```python
from build123d import *

# Parameters (mm, degrees)
SKETCH2_R          = 15
SKETCH2_R_2        = 8.75
M10_TAPPED_HOLE1_D = 8.5
M10_TAPPED_HOLE2_D = 8.5


with BuildPart() as part:
    # Sweep1: sweep along a path in Sketch1
    with BuildLine(Plane(origin=(0, 0, 0), x_dir=(1, 0, 0), z_dir=(0, 1, 0))) as sweep1_path:
        Line((175, 180), (175, 30))
        ThreePointArc((175, 30), (166.213203436, 8.786796564), (145, 0))
        Line((145, 0), (-145, 0))
        ThreePointArc((-145, 0), (-166.213203436, -8.786796564), (-175, -30))
        Line((-175, -30), (-175, -180))
    # Sketch2 → Sweep1 (sweep)
    with BuildSketch(Plane(origin=(0, 0, 0), x_dir=(0, 0, -1), z_dir=(1, 0, 0))):
        Circle(SKETCH2_R)
        Circle(SKETCH2_R_2, mode=Mode.SUBTRACT)
    sweep(path=sweep1_path.line)

    # M10 Tapped Hole1 (through all)
    with Locations(Plane(origin=(-190, 0, 145), x_dir=(0, -1, 0), z_dir=(-1, 0, 0))):
        with Locations((0, 0)):
            Hole(M10_TAPPED_HOLE1_D / 2)

    # M10 Tapped Hole2 (through all)
    with Locations(Plane(origin=(190, 0, -145), x_dir=(0, 0, 1), z_dir=(1, 0, 0))):
        with Locations((0, 0)):
            Hole(M10_TAPPED_HOLE2_D / 2)


solid = part.part
```
Geometry: final body of the model. Coordinates: model frame, mm. A direction names the side the tool comes from. Round coordinates to 2 decimals unless told otherwise and drop trailing zeros. Order: outer loops, then holes, each group sorted by start corner. A loop starts at its lowest first (then second) coordinate and runs counter-clockwise, first axis right, second up. Notation, with made-up numbers: (65.5, 54) -> (109.5, 54) arc R31 cw to (109.5, 79) -> close; hole circle Ø11 at (-3, 5). An arc over 180 degrees is marked (long way). Use CSV: the item, a comma, the result in double quotes. Start each with the question number.
1) Section A-A (z = -145). Return the cut outline in (x, y), and give its area (3 significant figures).
2) Section B-B (x = -21). Return the cut outline in (y, z), and give its area (3 significant figures).
3) First-contact query: pin 1 Ø8 at (x, y) = (-21, 6.5) entering from -Z; pin 2 Ø3 at (x, y) = (-120, 7.5) entering from +Z; pin 3 Ø6 at (y, z) = (8.5, 72) entering from -X. Flat tips, straight axial feed; report the tip coordinate or a pass-through.
4) Draft query along X for faces 4 (the face through (-183.346, -2.628, 106.05)), 5 (the face through (-160.015, -0.66, 106.05)), 6 (the face through (-163.622, -0.553, 149.214)). Return one class per face: +X half, -X half, draft (parallel to the pull), parting line (faces both ways), or undercut.
5) Material intervals for line 1 along Z through (x, y) = (42, 0); line 2 along X through (y, z) = (0, -120), sorted ascending. Write a range as from..to.
6) Section C-C (z = 74). Return the cut outline in (x, y), and give its area (3 significant figures).
7) Set-up query: faces 1 (the face through (166.654, -2.628, -103.95)), 2 (the face through (168.5, -6.5, -180)), 3 (the face through (-2.03, 14.643, 3.252)). Return all of +Z, -Z, +X, -X, +Y, -Y with unobstructed straight access to the full face (end or side cutting, diameter ignored); none if empty.
Returned:
1,outline,"(160.61, -4.25) arc R15 ccw to (189.39, -4.25) -> (182.65, -4.25) arc R8.75 cw to (167.35, -4.25) -> close; (160.61, 4.25) -> (167.35, 4.25) arc R8.75 cw to (182.65, 4.25) -> (189.39, 4.25) arc R15 ccw to start"
1,area,"357 mm²"
2,outline,"circle Ø30 at (0, 0); hole circle Ø17.5 at (0, 0)"
2,area,"466 mm²"
3,pin 1,"stops at z = -14.79"
3,pin 2,"stops at z = 13.75"
3,pin 3,"stops at x = -188.96"
4,face 4,"undercut"
4,face 5,"parting line"
4,face 6,"draft"
5,line 1,"z = -15..-8.75, 8.75..15"
5,line 2,"x = 160..166.25, 183.75..190"
6,outline,"circle Ø30 at (-175, 0); hole circle Ø17.5 at (-175, 0)"
6,area,"466 mm²"
7,face 1,"-Z"
7,face 2,"-Z, +X, -X, +Y, -Y"
7,face 3,"none"
